```python
from build123d import *

# Parameters (mm, degrees)
CUT_EXTRUDE1_REACH             = 38.532
CUT_EXTRUDE1_DIRECTION_2_REACH = 38.532
CHAMFER1_SIZE                  = 1
CHAMFER2_SIZE                  = 0.5
CHAMFER2_SIZE2                 = 0.288675135


with BuildPart() as part:
    # Sketch1 → Revolve1 (revolve)
    with BuildSketch(Plane.XY, mode=Mode.PRIVATE) as revolve1_sk:
        Polygon((-15.060768988, 23.176328976), (-19, 22.481736265), (-19, 19.651328976), (-10.35, -0.323671024), (-8.6, -0.323671024), (-8.6, -6.823671024), (-5.6, -6.823671024), (-5.6, 3.426328976), (-3, 3.426328976), (-3, -1.573671024), (0, -1.573671024), (0, 23.176328976), align=None)
    revolve(revolve1_sk.sketch.rotate(Axis((0, -1.573671024, 0), (0, 1, 0)), 270), axis=Axis((0, -1.573671024, 0), (0, 1, 0)))

    # Cut-Extrude1: up to this face of the body (flat: up to its plane)
    cut_extrude1_end = Plane(part.part.faces().sort_by_distance((0, 3.426328976, 5.441608081))[0])
    # Sketch3 → Cut-Extrude1 (cut, up to the picked face)
    with BuildSketch(Plane.XZ.offset(1.573671024), mode=Mode.PRIVATE) as cut_extrude1_sk1:
        Polygon((0.75, 1.85), (0, 1.1), (0, -1.1), (0.75, -1.85), (6.25, -1.85), (7, -1.1), (7, 1.1), (6.25, 1.85), align=None)
    cut_extrude1_tool1 = split(extrude(cut_extrude1_sk1.sketch, amount=-CUT_EXTRUDE1_REACH, mode=Mode.PRIVATE), bisect_by=cut_extrude1_end, keep=Keep.BOTH, mode=Mode.PRIVATE)
    add(cut_extrude1_tool1.solids().sort_by(Axis((3.5, -1.573671, 0), (0, 1, 0)))[0], mode=Mode.SUBTRACT)

    # Cut-Extrude1 direction 2: up to this face of the body (flat: up to its plane)
    cut_extrude1_direction_2_end = Plane(part.part.faces().sort_by_distance((0, -6.823671024, 8.356755267))[0])
    # Sketch3 → Cut-Extrude1 direction 2 (cut, up to the picked face)
    with BuildSketch(Plane.XZ.offset(1.573671024), mode=Mode.PRIVATE) as cut_extrude1_direction_2_sk1:
        Polygon((0.75, 1.85), (0, 1.1), (0, -1.1), (0.75, -1.85), (6.25, -1.85), (7, -1.1), (7, 1.1), (6.25, 1.85), align=None)
    cut_extrude1_direction_2_tool1 = split(extrude(cut_extrude1_direction_2_sk1.sketch, amount=CUT_EXTRUDE1_DIRECTION_2_REACH, mode=Mode.PRIVATE), bisect_by=cut_extrude1_direction_2_end, keep=Keep.BOTH, mode=Mode.PRIVATE)
    add(cut_extrude1_direction_2_tool1.solids().sort_by(Axis((3.5, -1.573671, 0), (0, -1, 0)))[0], mode=Mode.SUBTRACT)

    # Chamfer1
    chamfer1_edges = [part.edges().sort_by_distance(p)[0] for p in [
        (-5.6, -6.823671024, 0),
    ]]
    chamfer(chamfer1_edges, length=CHAMFER1_SIZE)

    # Chamfer2
    chamfer2_edges = [part.edges().sort_by_distance(p)[0] for p in [
        (0, -6.823671024, 8.6),
    ]]
    chamfer2_side = [part.faces().sort_by_distance(p)[0] for p in [
        (0, -3.573671024, 8.6),
    ]]
    chamfer(chamfer2_edges, length=CHAMFER2_SIZE, length2=CHAMFER2_SIZE2, reference=chamfer2_side[0])


solid = part.part
```
Check sheet for the modelled part. Datum: model origin and axes. Units: mm. A direction names the side the tool comes from. Give positions to 0.01 mm unless a question says otherwise; leave off trailing zeros. Loops run counter-clockwise (first coordinate to the right, second up) from the corner with the lowest first, then second, coordinate; pieces in that order, holes last. Notation, with made-up numbers: (68, 71) - (77, 71) arc R13 ccw to (77, 95) - close; hole circle Ø6 at (85, -31.75). An arc over 180 degrees is marked (long way). One line per question, with ' | ' between items. Start each with the question number.
1. Cross-section at B-B, the plane z = 0. Enter the section's corners in (x, y).
2. Cross-section at A-A, the plane y = -1. Enter the section's corners in (x, z).
3. Material ranges on line 1 along X through (y, z) = (1, 0); line 2 along X through (y, z) = (0, 0); line 3 along X through (y, z) = (-2, 0), recorded low to high. Write a range as [from, to].
4. Set-up check for faces 1 (the flat face through (2, 1, -1.85)), 2 (the cylindrical face through (11.56, 21.05, 15.08)): record each of +Z, -Z, +X, -X, +Y, -Y from which the full face is reachable in a straight line by a thin tool's end or side.
5. Draft check along Z on faces 3 (the flat face through (-1, -1.574, 0)), 4 (the conical face through (14.943, 23.133, 3.318)), 5 (the flat face through (-6, -6.824, -4)). Enter one of: released by +Z, released by -Z, zero draft, split by the parting line, or undercut.
6. Gauge pin test, flat ends, axial feed: pin 1 Ø1.3 at (x, y) = (1.5, 2) entering from -Z; pin 2 Ø4.5 at (x, z) = (-1.5, 1.5) entering from -Y; pin 3 Ø0.7 at (y, z) = (0.5, 0.5) entering from -X. Record the tip position at first contact, or that the pin passes through.
Check result:
1) outline: (-19, 19.65) - (-10.35, -0.32) - (-8.6, -0.32) - (-8.6, -6.32) - (-8.31, -6.82) - (-6.6, -6.82) - (-5.6, -5.82) - (-5.6, 3.43) - (-3, 3.43) - (-3, -1.57) - (0, -1.57) - (0, 3.43) - (7, 3.43) - (7, -6.82) - (8.31, -6.82) - (8.6, -6.32) - (8.6, -0.32) - (10.35, -0.32) - (19, 19.65) - (19, 22.48) - (15.06, 23.18) - (-15.06, 23.18) - (-19, 22.48) - close
2) outline: circle Ø17.2 at (0, 0); (0, -1.1) - (0, 1.1) - (0.75, 1.85) - (2.36, 1.85) arc R3 ccw (long way) to (2.36, -1.85) - (0.75, -1.85) - close; hole (5.29, -1.85) - (6.25, -1.85) - (7, -1.1) - (7, 1.1) - (6.25, 1.85) - (5.29, 1.85) arc R5.6 ccw (long way) to start
3) line 1: x = [-10.92, -5.6], [-3, 0], [7, 10.92] | line 2: x = [-10.49, -5.6], [-3, 0], [7, 10.49] | line 3: x = [-8.6, -5.6], [7, 8.6]
4) face 1: -Y | face 2: +Y, -Y
5) face 3: undercut | face 4: split by the parting line | face 5: zero draft
6) pin 1: stops at z = -11.55 | pin 2: stops at y = -1.57 | pin 3: stops at x = -10.85
